```python
from build123d import *

# Parameters (mm, degrees)
EXTRUDE1_DEPTH      = 7.62
SKETCH2_R           = 2.25
EXTRUDE2_DEPTH      = 7.62
SKETCH3_R           = 2.25
SKETCH3_R_2         = 2.5
EXTRUDE3_DEPTH      = 7.62
SKETCH5_R           = 19.05
EXTRUDE5_DEPTH      = 9.222
EXTRUDE7_DEPTH      = 68.4
FILLET1_R           = 2.54
CHAMFER1_SIZE       = 0.508
CHAMFER2_SIZE       = 0.508
SKETCH8_R           = 5.835393935
EXTRUDE9_DEPTH      = 2.54
CHAMFER6_SIZE       = 0.254
CHAMFER7_SIZE       = 0.508
CHAMFER8_SIZE       = 0.508
SKETCH9_R           = 4.7625
CUT_EXTRUDE1_DEPTH  = 2.54
SKETCH10_R          = 3.175
BOSS_EXTRUDE1_DEPTH = 20.94
BOSS_EXTRUDE2_START = 17.538
SKETCH11_R          = 3.175
BOSS_EXTRUDE2_DEPTH = 17.538
CHAMFER9_SIZE       = 0.254
CHAMFER10_SIZE      = 0.254
CHAMFER11_SIZE      = 0.254
SKETCH12_W          = 8.536855061
SKETCH12_H          = 3.479171119
CUT_EXTRUDE2_DEPTH  = 16
CHAMFER12_SIZE      = 0.1
SKETCH13_W          = 12.128390522
SKETCH13_H          = 4.389322284
CUT_EXTRUDE3_DEPTH  = 14
CHAMFER13_SIZE      = 0.1


with BuildPart() as part:
    # Sketch1 → Extrude1 (new body)
    with BuildSketch(Plane.XY):
        with BuildLine():
            Line((25.7, -28.2), (-25.7, -28.2))
            ThreePointArc((-25.7, -28.2), (-27.467766953, -27.467766953), (-28.2, -25.7))
            Line((-28.2, -25.7), (-28.2, 25.7))
            ThreePointArc((-28.2, 25.7), (-27.467766953, 27.467766953), (-25.7, 28.2))
            Line((-25.7, 28.2), (25.7, 28.2))
            ThreePointArc((25.7, 28.2), (27.467766953, 27.467766953), (28.2, 25.7))
            Line((28.2, 25.7), (28.2, -25.7))
            ThreePointArc((28.2, -25.7), (27.467766953, -27.467766953), (25.7, -28.2))
        make_face()
    extrude(amount=EXTRUDE1_DEPTH)

    # Sketch2 → Extrude2 (cut)
    with BuildSketch(Plane.XY.offset(7.62)):
        with Locations((-23.569999999, 23.57)):
            Circle(SKETCH2_R)
    extrude(amount=-EXTRUDE2_DEPTH, mode=Mode.SUBTRACT)

    # Sketch3 → Extrude3 (cut)
    with BuildSketch(Plane.XY.offset(7.62)):
        with Locations((23.569999999, 23.57)):
            Circle(SKETCH3_R)
        with Locations((23.569999999, -23.57)):
            Circle(SKETCH3_R)
        with Locations((-23.57, -23.57)):
            Circle(SKETCH3_R_2)
    extrude(amount=-EXTRUDE3_DEPTH, mode=Mode.SUBTRACT)

    # Sketch5 → Extrude5 (add)
    with BuildSketch(Plane.XY):
        Circle(SKETCH5_R)
    extrude(amount=EXTRUDE5_DEPTH)

    # Sketch6 → Extrude7 (add)
    with BuildSketch(Plane.XY):
        with BuildLine():
            Line((-18.94, 28.2), (-18.94, 23.57))
            ThreePointArc((-18.94, 23.57), (-20.296095603, 20.296095603), (-23.57, 18.94))
            Line((-23.57, 18.94), (-28.2, 18.94))
            Line((-28.2, 18.94), (-28.2, -18.939999999))
            Line((-28.2, -18.939999999), (-23.57, -18.939999999))
            ThreePointArc((-23.57, -18.939999999), (-20.296095603, -20.296095602), (-18.94, -23.569999999))
            Line((-18.94, -23.569999999), (-18.94, -28.2))
            Line((-18.94, -28.2), (-5.065990887, -28.2))
            Line((-5.065990887, -28.2), (5.065990887, -28.2))
            Line((5.065990887, -28.2), (18.939999999, -28.2))
            Line((18.939999999, -28.2), (18.939999999, -23.569999999))
            ThreePointArc((18.939999999, -23.569999999), (20.296095602, -20.296095602), (23.569999999, -18.939999999))
            Line((23.569999999, -18.939999999), (28.2, -18.939999999))
            Line((28.2, -18.939999999), (28.2, 18.94))
            Line((28.2, 18.94), (23.57, 18.94))
            ThreePointArc((23.57, 18.94), (20.296095602, 20.296095603), (18.939999999, 23.57))
            Line((18.939999999, 23.57), (18.939999999, 28.2))
            Line((18.939999999, 28.2), (-18.94, 28.2))
        make_face()
    extrude(amount=-EXTRUDE7_DEPTH)

    # Fillet1
    fillet1_edges = [part.edges().sort_by_distance(p)[0] for p in [
        (20.296095602, 20.296095603, -68.4),
        (18.939999999, 25.885, -68.4),
        (-1e-09, 28.2, -68.4),
        (-18.94, 25.885, -68.4),
        (-20.296095603, 20.296095603, -68.4),
        (-25.885, 18.94, -68.4),
        (-28.2, 0, -68.4),
        (-25.885, -18.939999999, -68.4),
        (-20.296095603, -20.296095602, -68.4),
        (-18.94, -25.885, -68.4),
        (-1e-09, -28.2, -68.4),
        (18.939999999, -25.885, -68.4),
        (20.296095602, -20.296095602, -68.4),
        (25.885, -18.939999999, -68.4),
        (28.2, 0, -68.4),
        (25.885, 18.94, -68.4),
        (18.939999999, -28.2, -34.2),
        (28.2, -18.939999999, -34.2),
        (-18.94, -28.2, -34.2),
        (-28.2, -18.939999999, -34.2),
        (28.2, 18.94, -34.2),
        (18.939999999, 28.2, -34.2),
        (-18.94, 28.2, -34.2),
        (-28.2, 18.94, -34.2),
    ]]
    fillet(fillet1_edges, radius=FILLET1_R)

    # Chamfer1
    chamfer1_edges = [part.edges().sort_by_distance(p)[0] for p in [
        (21.049999999, 28.2, 0),
        (27.467766953, 27.467766953, 0),
        (28.2, 21.05, 0),
    ]]
    chamfer(chamfer1_edges, length=CHAMFER1_SIZE)

    # Chamfer2
    chamfer2_edges = [part.edges().sort_by_distance(p)[0] for p in [
        (-28.2, -21.049999999, 0),
        (-21.05, -28.2, 0),
        (-27.467766953, -27.467766953, 0),
    ]]
    chamfer(chamfer2_edges, length=CHAMFER2_SIZE)

    # Sketch8 → Extrude9 (cut)
    with BuildSketch(Plane(origin=(0, 0, -68.4), x_dir=(-1, 0, 0), z_dir=(0, 0, -1))):
        Circle(SKETCH8_R)
    extrude(amount=-EXTRUDE9_DEPTH, mode=Mode.SUBTRACT)

    # Chamfer6
    chamfer6_edges = [part.edges().sort_by_distance(p)[0] for p in [
        (5.835393935, 0, -68.4),
    ]]
    chamfer(chamfer6_edges, length=CHAMFER6_SIZE)

    # Chamfer7
    chamfer7_edges = [part.edges().sort_by_distance(p)[0] for p in [
        (28.2, -21.049999999, 0),
        (27.467766953, -27.467766953, 0),
        (21.049999999, -28.2, 0),
    ]]
    chamfer(chamfer7_edges, length=CHAMFER7_SIZE)

    # Chamfer8
    chamfer8_edges = [part.edges().sort_by_distance(p)[0] for p in [
        (-27.467766953, 27.467766953, 0),
        (-28.2, 21.05, 0),
        (-21.05, 28.2, 0),
    ]]
    chamfer(chamfer8_edges, length=CHAMFER8_SIZE)

    # Sketch9 → Cut-Extrude1 (cut)
    with BuildSketch(Plane.XY.offset(9.222)):
        Circle(SKETCH9_R)
    extrude(amount=-CUT_EXTRUDE1_DEPTH, mode=Mode.SUBTRACT)

    # Sketch10 → Boss-Extrude1 (add)
    with BuildSketch(Plane.XY.offset(6.682)):
        Circle(SKETCH10_R)
    extrude(amount=BOSS_EXTRUDE1_DEPTH)

    # Sketch11 → Boss-Extrude2 (add)
    with BuildSketch(Plane(origin=(0, 0, -65.86), x_dir=(-1, 0, 0), z_dir=(0, 0, -1)).offset(BOSS_EXTRUDE2_START)):
        with Locations(Location((0, 0, 0), (0, 0, 180))):
            Circle(SKETCH11_R)
    extrude(amount=-BOSS_EXTRUDE2_DEPTH)

    # Chamfer9
    chamfer9_edges = [part.edges().sort_by_distance(p)[0] for p in [
        (-19.05, 0, 9.222),
    ]]
    chamfer(chamfer9_edges, length=CHAMFER9_SIZE)

    # Chamfer10
    chamfer10_edges = [part.edges().sort_by_distance(p)[0] for p in [
        (-25.819999999, 23.57, 7.62),
        (21.319999999, 23.57, 7.62),
        (-26.07, -23.57, 7.62),
        (21.319999999, -23.57, 7.62),
    ]]
    chamfer(chamfer10_edges, length=CHAMFER10_SIZE)

    # Chamfer11
    chamfer11_edges = [part.edges().sort_by_distance(p)[0] for p in [
        (-25.819999999, 23.57, 0),
        (21.319999999, 23.57, 0),
        (-26.07, -23.57, 0),
        (21.319999999, -23.57, 0),
    ]]
    chamfer(chamfer11_edges, length=CHAMFER11_SIZE)

    # Sketch12 → Cut-Extrude2 (cut)
    with BuildSketch(Plane.XY.offset(27.622)):
        with Locations((0.361580674, 4.36458556)):
            Rectangle(SKETCH12_W, SKETCH12_H)
    extrude(amount=-CUT_EXTRUDE2_DEPTH, mode=Mode.SUBTRACT)

    # Chamfer12
    chamfer12_edges = [part.edges().sort_by_distance(p)[0] for p in [
        (-1.48490634, -2.806363868, 27.622),
        (0, 2.625, 27.622),
        (0, 3.175, 11.622),
    ]]
    chamfer(chamfer12_edges, length=CHAMFER12_SIZE)

    # Sketch13 → Cut-Extrude3 (cut)
    with BuildSketch(Plane(origin=(0, 0, -83.398), x_dir=(-1, 0, 0), z_dir=(0, 0, -1))):
        with Locations((0.157033553, 4.819661142)):
            Rectangle(SKETCH13_W, SKETCH13_H)
    extrude(amount=-CUT_EXTRUDE3_DEPTH, mode=Mode.SUBTRACT)

    # Chamfer13
    chamfer13_edges = [part.edges().sort_by_distance(p)[0] for p in [
        (-1.48490634, -2.806363868, -83.398),
        (0, 2.625, -83.398),
        (0, 3.175, -69.398),
    ]]
    chamfer(chamfer13_edges, length=CHAMFER13_SIZE)


solid = part.part
```
Model file for the job. Use its own axes, mm. A direction names the side the tool comes from. Give positions to 0.01 mm unless a question says otherwise; leave off trailing zeros. Write each loop counter-clockwise with the first axis right and the second up, starting at its lowest first coordinate (ties: lowest second). Pieces come first, ordered by that corner, then holes. Notation, with made-up numbers: (72.5, -18.75) -> (90.5, -18.75) arc R16 cw to (90.5, -0.75) -> close; hole circle Ø8 at (63.5, 22). An arc over 180 degrees is marked (long way). Use CSV: the item, a comma, the result in double quotes. Start each with the question number.
1) Tool access for faces 1 (the flat face through (25, -18.94, -32)), 2 (the cylindrical face through (-27.476, 18.176, -33.141)), 3 (the cylindrical face through (-5.566, 1.753, -67.019)): list every direction of +Z, -Z, +X, -X, +Y, -Y with a clear straight run to the whole face (end or side of a thin tool).
2) Cut at A-A on z = -59.5. List the corners of the cut face in (x, y), plus the area to 3 significant figures.
3) Pin check, flat tips, straight feed: P1, Ø3.5, axis at x = -23.57, y = 23.57, coming from the -Z side; P2, Ø7, axis at x = 23.57, y = 23.57, coming from the -Z side; P3, Ø2.5, axis at x = 24, z = -19, coming from the +Y side; P4, Ø1.7, axis at x = 25, z = -42, coming from the -Y side. Stop position of each tip, or through.
4) Drill centre lines: L1, parallel to Y at x = -23.57, z = 2; L2, parallel to Y at x = -23, z = 4; L3, parallel to X at y = 23, z = 4. Where is each one in solid material? Low to high.
5) Two-plate mould, pull along Y, no slides. Class faces 4 (the cylindrical face through (-27.436, -0.23, -67.676)), 5 (the cylindrical face through (-3.78, -2.9, 7.97)), 6 (the flat face through (0, -28.2, -30)): released by +Y, released by -Y, zero draft, split by the parting line, or undercut.
Final values:
1,face 1,"-Z, +X, -Y"
1,face 2,"-Z, -X, +Y"
1,face 3,"-Z"
2,outline,"(-28.2, -16.4) arc R2.54 ccw to (-25.66, -18.94) -> (-23.57, -18.94) arc R4.63 cw to (-18.94, -23.57) -> (-18.94, -25.66) arc R2.54 ccw to (-16.4, -28.2) -> (16.4, -28.2) arc R2.54 ccw to (18.94, -25.66) -> (18.94, -23.57) arc R4.63 cw to (23.57, -18.94) -> (25.66, -18.94) arc R2.54 ccw to (28.2, -16.4) -> (28.2, 16.4) arc R2.54 ccw to (25.66, 18.94) -> (23.57, 18.94) arc R4.63 cw to (18.94, 23.57) -> (18.94, 25.66) arc R2.54 ccw to (16.4, 28.2) -> (-16.4, 28.2) arc R2.54 ccw to (-18.94, 25.66) -> (-18.94, 23.57) arc R4.63 cw to (-23.57, 18.94) -> (-25.66, 18.94) arc R2.54 ccw to (-28.2, 16.4) -> close"
2,area,"2,850 mm2"
3,P1,"passes through"
3,P2,"stops at z = 0"
3,P3,"stops at y = 19.01"
3,P4,"stops at y = -18.94"
4,L1,"y = -28.2 to -26.07, -21.07 to 21.32, 25.82 to 28.2"
4,L2,"y = -28.2 to -26, -21.14 to 21.39, 25.75 to 28.2"
4,L3,"x = -28.2 to -25.75, -21.39 to 21.39, 25.75 to 28.2"
5,face 4,"zero draft"
5,face 5,"undercut"
5,face 6,"released by -Y"
